```python
from build123d import *

# Parameters (mm, degrees)
F0_W     = 76.2
F0_H     = 76.2
F1_DEPTH = 152.4
F2_W     = 36.068
F2_H     = 8.001
F3_DEPTH = 152.401
F4_W     = 3.175
F4_H     = 4.0005
F5_DEPTH = 152.401
F6_W     = 36.83
F6_H     = 68.199
F7_DEPTH = 50.8


with BuildPart() as f1:
    # F0 (on Right) → F1 (new body)
    with BuildSketch(Plane.YZ):
        with Locations((38.1, 38.1)):
            Rectangle(F0_W, F0_H)
    extrude(amount=F1_DEPTH)

    # F2 (on face) → F3 (cut, through all)
    with BuildSketch(Plane.YZ.offset(152.4)):
        with Locations((38.1, 72.1995)):
            Rectangle(F2_W, F2_H)
    extrude(amount=-F3_DEPTH, mode=Mode.SUBTRACT)

    # F4 (on face) → F5 (cut, through all)
    with BuildSketch(Plane.YZ.offset(152.4)):
        with Locations((18.4785, 74.19975)):
            Rectangle(F4_W, F4_H)
        with Locations((57.7215, 74.19975)):
            Rectangle(F4_W, F4_H)
    extrude(amount=-F5_DEPTH, mode=Mode.SUBTRACT)

    # F6 (on face) → F7 (cut)
    with BuildSketch(Plane(origin=(0, 0, 0), x_dir=(0, -1, 0), z_dir=(-1, 0, 0))):
        with Locations((-38.1, 34.0995)):
            Rectangle(F6_W, F6_H)
    extrude(amount=-F7_DEPTH, mode=Mode.SUBTRACT)


solid = f1.part
```
For this review, take the finished solid that the model builds, in its own axes (mm). A direction names the side the tool comes from. Coordinates: 2 decimals unless noted, no trailing zeros. Loops run counter-clockwise (first coordinate to the right, second up) from the corner with the lowest first, then second, coordinate; pieces in that order, holes last.
1. Add section D-D, the plane y = 33. Give the boundary of the cut face in (x, z).
2. For faces 5 (the flat face through (77, 20.066, 70)), 6 (the flat face through (75, 8, 76.2)), 7 (the flat face through (25, 56.515, 34)), list the 3-axis set-ups (+Z, -Z, +X, -X, +Y, -Y) from which the entire face can be reached by the end or side of a thin tool; tool diameter is ignored.
3. For line 1 (Y direction, x = 33.5, z = 59.5) (3 decimals); line 2 (Z direction, x = 83, y = 28); line 3 (X direction, y = 52.5, z = 33), list the stretches that pass through material, from the lowest coordinate up.
4. Add section C-C, the plane x = 85.5. Give the boundary of the cut face in (y, z).
5. Mouldability with a two-part tool opening along Y and no side actions: class faces 1 (the flat face through (75, 68, 76.2)), 2 (the flat face through (75, 0, 38)), 3 (the flat face through (75, 76.2, 38)), 4 (the flat face through (77, 59.309, 74)) as +Y half, -Y half, draft (parallel to the pull), parting line (faces both ways), or undercut.
6. Add section B-B, the plane z = 9.5. Give the boundary of the cut face in (x, y) (3 decimals), then the cut area to 3 significant figures.
7. Insertion check: P1, Ø6, axis at x = 87.5, z = 63, coming from the -Y side; P2, Ø4, axis at y = 33, z = 32, coming from the -X side; P3, Ø3.5, axis at x = 96.5, y = 57.5, coming from the +Z side. Each pin has a flat end and moves straight along its axis. Give the tip position at first contact, or say it passes through.
Result:
1. outline: (50.8, 0) - (152.4, 0) - (152.4, 68.2) - (50.8, 68.2) - close
2. face 5: +Z, +X, -X
2. face 6: +Z, +X, -X, +Y, -Y
2. face 7: -Z, -X
3. line 1: y = 0 to 19.685, 56.515 to 76.2
3. line 2: z = 0 to 68.2
3. line 3: x = 50.8 to 152.4
4. outline: (0, 0) - (76.2, 0) - (76.2, 76.2) - (59.31, 76.2) - (59.31, 72.2) - (56.13, 72.2) - (56.13, 68.2) - (20.07, 68.2) - (20.07, 72.2) - (16.89, 72.2) - (16.89, 76.2) - (0, 76.2) - close
5. face 1: draft
5. face 2: -Y half
5. face 3: +Y half
5. face 4: undercut
6. outline: (0, 0) - (152.4, 0) - (152.4, 76.2) - (0, 76.2) - (0, 56.515) - (50.8, 56.515) - (50.8, 19.685) - (0, 19.685) - close
6. area: 9,740 mm2
7. P1: stops at y = 0
7. P2: stops at x = 50.8
7. P3: stops at z = 72.2
